```python
from build123d import *

# Parameters (mm, degrees)
SKETCH1_R           = 7.5
SKETCH1_R_2         = 5
BOSS_EXTRUDE1_DEPTH = 1
SKETCH2_R           = 6.5
SKETCH2_R_2         = 5
BOSS_EXTRUDE2_DEPTH = 3.5
CHAMFER1_SIZE       = 1


with BuildPart() as part:
    # Sketch1 → Boss-Extrude1 (new body)
    with BuildSketch(Plane.XY):
        Circle(SKETCH1_R)
        Circle(SKETCH1_R_2, mode=Mode.SUBTRACT)
    extrude(amount=BOSS_EXTRUDE1_DEPTH)

    # Sketch2 → Boss-Extrude2 (add)
    with BuildSketch(Plane.XY.offset(1)):
        Circle(SKETCH2_R)
        Circle(SKETCH2_R_2, mode=Mode.SUBTRACT)
    extrude(amount=BOSS_EXTRUDE2_DEPTH)

    # Chamfer1
    chamfer1_edges = [part.edges().sort_by_distance(p)[0] for p in [
        (-6.5, 0, 1),
    ]]
    chamfer(chamfer1_edges, length=CHAMFER1_SIZE - 0.0001)  # a hair under: the kernel refuses the full size

    # Mirror5: part across plane


with BuildPart() as part_1:
    add(part.part)
    add(part.part.mirror(Plane.XY.offset(4.5)))


solid = part_1.part
```
Read the model definition and answer for the solid it produces. Units are mm, in the model's axes. Give positions to 0.01 mm unless a question says otherwise; leave off trailing zeros. Order: outer loops, then holes, each group sorted by start corner. A loop starts at its lowest first (then second) coordinate and runs counter-clockwise, first axis right, second up.
(1) Straight lines are drawn through the part: L1, parallel to Y at x = 0, z = 6.2; L2, parallel to Z at x = -2.75, y = 6; L3, parallel to Y at x = -2.5, z = 3.25. For each, find the intervals that lie inside material, in ascending order.
(2) Given pin 1 (1 mm diameter, centred on y = 5, z = 5.5, fed in from +X); pin 2 (1 mm diameter, centred on x = 0.5, z = 5, fed in from +Y); pin 3 (3 mm diameter, centred on x = 0.5, z = 3, fed in from +Y), each flat-ended and moving along its own axis, determine where each tip first touches the part or whether it passes through.
(3) Find section C-C (z = 5.25). Give the vertices of the cut face in (x, y).
Result sheet:
1. L1: y = -6.5 to -5, 5 to 6.5
1. L2: z = 0 to 1.9, 7.1 to 9
1. L3: y = -6 to -4.33, 4.33 to 6
2. pin 1: stops at x = 4.69
2. pin 2: stops at y = 6.5
2. pin 3: stops at y = 6.99
3. outline: circle Ø13 at (0, 0); hole circle Ø10 at (0, 0)
